from build123d import *

# Parameters (mm, degrees)
SKETCH3_W           = 234.95
SKETCH3_H           = 76
SKETCH3_R           = 1.5
BOSS_EXTRUDE4_DEPTH = 3
SKETCH4_W           = 215.9
SKETCH4_H           = 12.7
CUT_EXTRUDE1_DEPTH  = 3.81
FILLET11_R          = 2.54


with BuildPart() as part:
    # Sketch3 → Boss-Extrude4 (new body)
    with BuildSketch(Plane(origin=(0, 0, 0), x_dir=(1, 0, 0), z_dir=(0, 1, 0))):
        with Locations((-117.475, -38)):
            Rectangle(SKETCH3_W, SKETCH3_H)
        with Locations(Location((-5.08, -3, 0), (0, 0, 270))):
            Circle(SKETCH3_R, mode=Mode.SUBTRACT)
        with Locations(Location((-5.08, -73, 0), (0, 0, 270))):
            Circle(SKETCH3_R, mode=Mode.SUBTRACT)
        with Locations(Location((-229.87, -73, 0), (0, 0, 270))):
            Circle(SKETCH3_R, mode=Mode.SUBTRACT)
        with Locations(Location((-229.87, -3, 0), (0, 0, 270))):
            Circle(SKETCH3_R, mode=Mode.SUBTRACT)
    extrude(amount=BOSS_EXTRUDE4_DEPTH)

    # Sketch4 → Cut-Extrude1 (cut)
    with BuildSketch(Plane(origin=(0, 3, 0), x_dir=(1, 0, 0), z_dir=(0, 1, 0))):
        with Locations((-117.475, -38)):
            Rectangle(SKETCH4_W, SKETCH4_H)
    extrude(amount=-CUT_EXTRUDE1_DEPTH, mode=Mode.SUBTRACT)

    # Fillet11
    fillet11_edges = [part.edges().sort_by_distance(p)[0] for p in [
        (-234.95, 1.5, 0),
        (0, 1.5, 0),
        (0, 1.5, 76),
        (-234.95, 1.5, 76),
    ]]
    fillet(fillet11_edges, radius=FILLET11_R)


solid = part.part
Input: part model. Units: mm. Frame: model coordinates. Coordinates: 2 decimals unless noted, no trailing zeros. Loops run counter-clockwise (first coordinate to the right, second up) from the corner with the lowest first, then second, coordinate; pieces in that order, holes last. Notation, with made-up numbers: (11, 57.25) - (38, 57.25) arc R26 ccw to (38, 87.25) - close; hole circle Ø2 at (35.5, 56). An arc over 180 degrees is marked (long way). Answer in a Markdown table with one row per item. Add a question column.
Item 1: Section query B-B on y = 0.75. Return the cut outline in (x, z) (3 decimals).
Item 2: Section query A-A on x = -171. Return the cut outline in (y, z), then the cut area to 3 significant figures.
Item 3: Line query: line 1 along Z through (x, y) = (-229.87, 1.7); line 2 along X through (y, z) = (2.1, 73); line 3 along Z through (x, y) = (-19.5, 2.6). Output: solid intervals per line, ascending. Write a range as [from, to].
Item 4: Contact query for a flat-ended pin moving along its axis: P1, Ø1.8, axis at x = -5.08, z = 3, coming from the -Y side. Output: stop coordinate, or through.
Recorded:
| question | item | result |
|---|---|---|
| 1 | outline | (-234.95, 2.54) arc R2.54 ccw to (-232.41, 0) - (-2.54, 0) arc R2.54 ccw to (0, 2.54) - (0, 73.46) arc R2.54 ccw to (-2.54, 76) - (-232.41, 76) arc R2.54 ccw to (-234.95, 73.46) - close; hole circle Ø3 at (-229.87, 3); hole circle Ø3 at (-229.87, 73); hole (-225.425, 31.65) - (-9.525, 31.65) - (-9.525, 44.35) - (-225.425, 44.35) - close; hole circle Ø3 at (-5.08, 3); hole circle Ø3 at (-5.08, 73) |
| 2 | outline | (0, 0) - (3, 0) - (3, 31.65) - (0, 31.65) - close; (0, 44.35) - (3, 44.35) - (3, 76) - (0, 76) - close |
| 2 | area | 190 mm^2 |
| 3 | line 1 | [0, 1.5], [4.5, 71.5], [74.5, 76] |
| 3 | line 2 | [-234.95, -231.37], [-228.37, -6.58], [-3.58, 0] |
| 3 | line 3 | [0, 31.65], [44.35, 76] |
| 4 | P1 | through |
